Autodesk Inventor part; units mm, degrees
ref_plane "YZ Plane" through (0, 0, 0) normal (1, 0, 0) x (0, 1, 0)
ref_plane "XZ Plane" through (0, 0, 0) normal (0, 1, 0) x (-1, 0, 0)
ref_plane "XY Plane" through (0, 0, 0) normal (0, 0, 1) x (1, 0, 0)
sketch "Sketch1" plane through (0, 0, 0) normal (1, 0, 0) x (0, 1, 0)
  circle A0 centre (0, 0) radius 7.5
  dimension "d0" = 15
extrude "Extrusion1" add sketch "Sketch1" along normal blind 60
sketch "Sketch2" plane through (60, 0, 0) normal (1, 0, 0) x (0, 0, -1)
  circle A0 centre (0, 0) radius 9
  dimension "d5" = 18
extrude "Extrusion2" add sketch "Sketch2" against normal blind 20
chamfer "Chamfer1" distance 2 angle 45 1 edges at (60, 0, 9)
chamfer "Chamfer2" distance 1 angle 45 1 edges at (40, 0, 9)
properties part number "Enbolo"
The listing builds one solid part. Answer for the finished solid, in the listing's coordinates (mm). A direction names the side the tool comes from. Round coordinates to 2 decimals unless told otherwise and drop trailing zeros. Loops run counter-clockwise (first coordinate to the right, second up) from the corner with the lowest first, then second, coordinate; pieces in that order, holes last. Notation, with made-up numbers: M -20,-0.75 L 22,-0.75 A12 cw 22,7.25 Z; hole C 33.25,89 d7. An arc over 180 degrees is marked long. Return JSON: item names as keys, results as strings.
Q1. Which of the six approach directions +Z, -Z, +X, -X, +Y, -Y give full straight-line access (tool end or side, diameter ignored) to faces 1 (the face through (19.72, -7.493, -0.33)), 2 (the face through (60, 0, 0))?
Results list:
{"face 1": "-X", "face 2": "+Z, -Z, +X, +Y, -Y"}
Q2. Each of these flat-tipped pins is pushed along its axis until it touches: pin 1 Ø3 at (x, z) = (19.5, -3.5) entering from +Y; pin 2 Ø3 at (x, z) = (26.5, 2) entering from +Y; pin 3 Ø3 at (x, y) = (24.5, 4.5) entering from +Z. Where does it stop, or does it pass through?
Results list:
{"pin 1": "stops at y = 7.23", "pin 2": "stops at y = 7.48", "pin 3": "stops at z = 6.87"}
Q3. Find section C-C, the plane x = 15. Determine the outline of the cut face in (y, z), plus the area to 3 significant figures.
Results list:
{"outline": "C 0,0 d15", "area": "177 mm2"}
Q4. Find the intervals of material crossed by line 1 along Y through (x, z) = (19, -2); line 2 along Y through (x, z) = (30, -0.25); line 3 along X through (y, z) = (6.25, 5.5), in increasing order. Write a range as from..to.
Results list:
{"line 1": "y = -7.23..7.23", "line 2": "y = -7.5..7.5", "line 3": "x = 40.33..58.67"}
Q5. Find section A-A, the plane z = 0. Determine the outline of the cut face in (x, y).
Results list:
{"outline": "M 0,-7.5 L 40,-7.5 L 40,-8 L 41,-9 L 58,-9 L 60,-7 L 60,7 L 58,9 L 41,9 L 40,8 L 40,7.5 L 0,7.5 Z"}
Q6. Find section D-D, the plane x = 43. Determine the outline of the cut face in (y, z).
Results list:
{"outline": "C 0,0 d18"}
